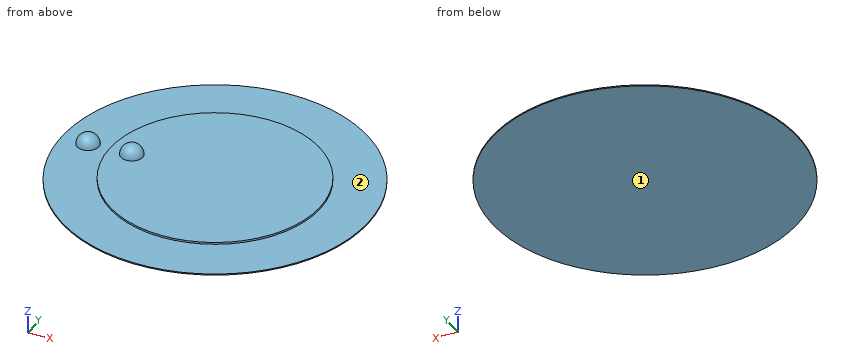
Autodesk Inventor part; units mm, degrees
ref_plane "YZ Plane" through (0, 0, 0) normal (1, 0, 0) x (0, 1, 0)
ref_plane "XZ Plane" through (0, 0, 0) normal (0, 1, 0) x (-1, 0, 0)
ref_plane "XY Plane" through (0, 0, 0) normal (0, 0, 1) x (1, 0, 0)
sketch "Sketch1" plane through (0, 0, 0) normal (0, 0, 1) x (1, 0, 0)
  circle A0 centre (0, 0) radius 17.5
  dimension "d0" = 35
extrude "Extrusion1" add sketch "Sketch1" along normal blind 0.13
sketch "Sketch2" plane through (0, 0, 0.13) normal (0, 0, 1) x (1, 0, 0)
  circle A0 centre (0, 0) radius 12
  dimension "d3" = 24
extrude "Extrusion2" add sketch "Sketch2" along normal blind 0.22
sketch "Sketch3" plane through (0, 0, 0.13) normal (0, 0, 1) x (1, 0, 0)
  circle A0 centre (0, 0) radius 17.5
  line L0 (-17.5, 0) -> (-14.5, 0)
  circle A1 centre (-14.5, 0) radius 1.25
  line L1 (-14.5, 0) -> (-13.25, 0)
  point P0 (-15.75, 0)
  dimension "d7" = 2.5
  dimension "d6" = 3
revolve "Revolution1" add sketch "Sketch3" angle 180 about axis through (-17.5, 0, 0.13) along (1, 0, 0) picked at (-14.1156, 0.7325) contours A1 L1 L0
sketch "Sketch4" plane through (0, 0, 0.35) normal (0, 0, 1) x (1, 0, 0)
  circle A0 centre (-14.5, 0) radius 1.25
  circle A1 centre (0, 0) radius 12
  circle A2 centre (0, 0) radius 17.5
  circle A3 centre (0, 0) radius 17.5
  line L0 (-17.5, 0) -> (-9.5, 0)
  circle A4 centre (-9.5, 0) radius 1.25
  line L1 (-9.5, 0) -> (-8.25, 0)
  point P0 (-10.75, 0)
  dimension "d10" = 2.5
  dimension "d9" = 8
revolve "Revolution2" add sketch "Sketch4" angle 180 about axis through (-17.5, 0, 0.35) along (1, 0, 0) picked at (-9.1156, 0.7325) contours A4 L1 L0
properties part number "Piezo"
Geometry check sheet. Reference: the model listing, model coordinates, mm. Face numbers are marked on the shaded views. A direction names the side the tool comes from. Coordinates: 2 decimals unless noted, no trailing zeros. Order: outer loops, then holes, each group sorted by start corner. A loop starts at its lowest first (then second) coordinate and runs counter-clockwise, first axis right, second up.
Item 1: Section check A-A (y = 0). Enter the section's corners in (x, z), plus the area to 3 significant figures.
Item 2: Section check B-B (x = 0). Enter the section's corners in (y, z).
Item 3: Tool access check on the marked faces 1 and 2. Record the directions out of +Z, -Z, +X, -X, +Y, -Y that give a thin tool (end or side, any length) a straight path to the whole face; none if there is none.
Item 4: Depth check by flat-ended pin: pin 1 (8 mm diameter, centred on x = 13, y = 13.5, fed in from +Z); pin 2 (10 mm diameter, centred on x = -5.5, y = 8.5, fed in from +Z); pin 3 (1.5 mm diameter, centred on x = -8.5, y = 3.5, fed in from -Z). Enter the tip coordinate at first touch or a pass-through.
Item 5: Scan lines: line 1 along Z through (x, y) = (5, 6.5); line 2 along Y through (x, z) = (-9.5, 0.4); line 3 along Y through (x, z) = (6.5, 0.3). Record each from-to range of solid material in increasing order.
Item 6: Section check D-D (x = 9.5). Enter the section's corners in (y, z), plus the area to 3 significant figures.
Item 7: Section check C-C (z = 0.65). Enter the section's corners in (x, y), plus the area to 3 significant figures.
Check sheet entries:
1. outline: (-17.5, 0) - (17.5, 0) - (17.5, 0.13) - (12, 0.13) - (12, 0.35) - (-8.25, 0.35) arc R1.25 ccw to (-10.75, 0.35) - (-12, 0.35) - (-12, 0.13) - (-13.25, 0.13) arc R1.25 ccw to (-15.75, 0.13) - (-17.5, 0.13) - close
1. area: 14.7 mm2
2. outline: (-17.5, 0) - (17.5, 0) - (17.5, 0.13) - (12, 0.13) - (12, 0.35) - (-12, 0.35) - (-12, 0.13) - (-17.5, 0.13) - close
3. face 1: -Z, +X, -X, +Y, -Y
3. face 2: +Z
4. pin 1: stops at z = 0.13
4. pin 2: stops at z = 0.35
4. pin 3: stops at z = 0
5. line 1: z = 0 to 0.35
5. line 2: y = -1.25 to 1.25
5. line 3: y = -10.09 to 10.09
6. outline: (-14.7, 0) - (14.7, 0) - (14.7, 0.13) - (7.33, 0.13) - (7.33, 0.35) - (-7.33, 0.35) - (-7.33, 0.13) - (-14.7, 0.13) - close
6. area: 7.05 mm2
7. outline: circle Ø2.27 at (-14.5, 0); circle Ø2.43 at (-9.5, 0)
7. area: 8.69 mm2
